from build123d import *

# Parameters (mm, degrees)
F1_DEPTH = 10
F2_START = 10
F2_DEPTH = 10
F3_START = 20
F3_DEPTH = 15
F4_START = 35
F4_DEPTH = 20


with BuildPart() as f1:
    # F0 (on Front) → F1 (new body)
    with BuildSketch(Plane.XZ):
        with BuildLine():
            Line((1.12e-08, 3), (-35, 3))
            Line((-35, 3), (-35, 0.5))
            Line((-35, 0.5), (-2.9580398915, 0.5))
            ThreePointArc((-2.9580398915, 0.5), (-1.9364916688, 2.2912878511), (1.12e-08, 3))
        make_face()
        with BuildLine():
            Line((-2.9580398915, 0.5), (-35, 0.5))
            Line((-35, 0.5), (-35, -0.5))
            Line((-35, -0.5), (-2.9580398915, -0.5))
            ThreePointArc((-2.9580398915, -0.5), (-3, 0), (-2.9580398915, 0.5))
        make_face()
        with BuildLine():
            Line((-2.9580398915, -0.5), (-35, -0.5))
            Line((-35, -0.5), (-35, -3))
            Line((-35, -3), (1.44e-08, -3))
            ThreePointArc((1.44e-08, -3), (-1.9364916676, -2.2912878521), (-2.9580398915, -0.5))
        make_face()
        with BuildLine():
            Line((2.9580398915, -0.5), (-2.9580398915, -0.5))
            ThreePointArc((-2.9580398915, -0.5), (-1.9364916676, -2.2912878521), (1.44e-08, -3))
            ThreePointArc((1.44e-08, -3), (1.9364916786, -2.2912878428), (2.9580398915, -0.5))
        make_face()
        with BuildLine():
            ThreePointArc((2.9580398915, 0.5), (1.9364916774, 2.2912878439), (1.12e-08, 3))
            ThreePointArc((1.12e-08, 3), (-1.9364916688, 2.2912878511), (-2.9580398915, 0.5))
            Line((-2.9580398915, 0.5), (2.9580398915, 0.5))
        make_face()
        with BuildLine():
            Line((35, 3), (1.12e-08, 3))
            ThreePointArc((1.12e-08, 3), (1.9364916774, 2.2912878439), (2.9580398915, 0.5))
            Line((2.9580398915, 0.5), (35, 0.5))
            Line((35, 0.5), (35, 3))
        make_face()
        with BuildLine():
            Line((35, 0.5), (2.9580398915, 0.5))
            ThreePointArc((2.9580398915, 0.5), (2.9894915684, 0.2508787808), (3, 0))
            ThreePointArc((3, 0), (2.9894915684, -0.2508787808), (2.9580398915, -0.5))
            Line((2.9580398915, -0.5), (35, -0.5))
            Line((35, -0.5), (35, 0.5))
        make_face()
        with BuildLine():
            Line((35, -3), (35, -0.5))
            Line((35, -0.5), (2.9580398915, -0.5))
            ThreePointArc((2.9580398915, -0.5), (1.9364916786, -2.2912878428), (1.44e-08, -3))
            Line((1.44e-08, -3), (35, -3))
        make_face()
        with BuildLine():
            ThreePointArc((3, 0), (2.9894915684, 0.2508787808), (2.9580398915, 0.5))
            Line((2.9580398915, 0.5), (-2.9580398915, 0.5))
            ThreePointArc((-2.9580398915, 0.5), (-3, 0), (-2.9580398915, -0.5))
            Line((-2.9580398915, -0.5), (2.9580398915, -0.5))
            ThreePointArc((2.9580398915, -0.5), (2.9894915684, -0.2508787808), (3, 0))
        make_face()
    extrude(amount=F1_DEPTH)

    # F0 (on Front) → F2 (join)
    with BuildSketch(Plane.XZ.offset(F2_START)):
        with BuildLine():
            Line((-2.9580398915, 0.5), (-35, 0.5))
            Line((-35, 0.5), (-35, -0.5))
            Line((-35, -0.5), (-2.9580398915, -0.5))
            ThreePointArc((-2.9580398915, -0.5), (-3, 0), (-2.9580398915, 0.5))
        make_face()
        with BuildLine():
            ThreePointArc((3, 0), (2.9894915684, 0.2508787808), (2.9580398915, 0.5))
            Line((2.9580398915, 0.5), (-2.9580398915, 0.5))
            ThreePointArc((-2.9580398915, 0.5), (-3, 0), (-2.9580398915, -0.5))
            Line((-2.9580398915, -0.5), (2.9580398915, -0.5))
            ThreePointArc((2.9580398915, -0.5), (2.9894915684, -0.2508787808), (3, 0))
        make_face()
        with BuildLine():
            Line((35, 0.5), (2.9580398915, 0.5))
            ThreePointArc((2.9580398915, 0.5), (2.9894915684, 0.2508787808), (3, 0))
            ThreePointArc((3, 0), (2.9894915684, -0.2508787808), (2.9580398915, -0.5))
            Line((2.9580398915, -0.5), (35, -0.5))
            Line((35, -0.5), (35, 0.5))
        make_face()
    extrude(amount=F2_DEPTH)

    # F0 (on Front) → F3 (join)
    with BuildSketch(Plane.XZ.offset(F3_START)):
        with BuildLine():
            Line((35, 3), (1.12e-08, 3))
            ThreePointArc((1.12e-08, 3), (1.9364916774, 2.2912878439), (2.9580398915, 0.5))
            Line((2.9580398915, 0.5), (35, 0.5))
            Line((35, 0.5), (35, 3))
        make_face()
        with BuildLine():
            Line((35, 0.5), (2.9580398915, 0.5))
            ThreePointArc((2.9580398915, 0.5), (2.9894915684, 0.2508787808), (3, 0))
            ThreePointArc((3, 0), (2.9894915684, -0.2508787808), (2.9580398915, -0.5))
            Line((2.9580398915, -0.5), (35, -0.5))
            Line((35, -0.5), (35, 0.5))
        make_face()
        with BuildLine():
            Line((35, -3), (35, -0.5))
            Line((35, -0.5), (2.9580398915, -0.5))
            ThreePointArc((2.9580398915, -0.5), (1.9364916786, -2.2912878428), (1.44e-08, -3))
            Line((1.44e-08, -3), (35, -3))
        make_face()
        with BuildLine():
            Line((-2.9580398915, -0.5), (-35, -0.5))
            Line((-35, -0.5), (-35, -3))
            Line((-35, -3), (1.44e-08, -3))
            ThreePointArc((1.44e-08, -3), (-1.9364916676, -2.2912878521), (-2.9580398915, -0.5))
        make_face()
        with BuildLine():
            Line((1.12e-08, 3), (-35, 3))
            Line((-35, 3), (-35, 0.5))
            Line((-35, 0.5), (-2.9580398915, 0.5))
            ThreePointArc((-2.9580398915, 0.5), (-1.9364916688, 2.2912878511), (1.12e-08, 3))
        make_face()
        with BuildLine():
            Line((-2.9580398915, 0.5), (-35, 0.5))
            Line((-35, 0.5), (-35, -0.5))
            Line((-35, -0.5), (-2.9580398915, -0.5))
            ThreePointArc((-2.9580398915, -0.5), (-3, 0), (-2.9580398915, 0.5))
        make_face()
        with BuildLine():
            ThreePointArc((2.9580398915, 0.5), (1.9364916774, 2.2912878439), (1.12e-08, 3))
            ThreePointArc((1.12e-08, 3), (-1.9364916688, 2.2912878511), (-2.9580398915, 0.5))
            Line((-2.9580398915, 0.5), (2.9580398915, 0.5))
        make_face()
        with BuildLine():
            ThreePointArc((3, 0), (2.9894915684, 0.2508787808), (2.9580398915, 0.5))
            Line((2.9580398915, 0.5), (-2.9580398915, 0.5))
            ThreePointArc((-2.9580398915, 0.5), (-3, 0), (-2.9580398915, -0.5))
            Line((-2.9580398915, -0.5), (2.9580398915, -0.5))
            ThreePointArc((2.9580398915, -0.5), (2.9894915684, -0.2508787808), (3, 0))
        make_face()
        with BuildLine():
            Line((2.9580398915, -0.5), (-2.9580398915, -0.5))
            ThreePointArc((-2.9580398915, -0.5), (-1.9364916676, -2.2912878521), (1.44e-08, -3))
            ThreePointArc((1.44e-08, -3), (1.9364916786, -2.2912878428), (2.9580398915, -0.5))
        make_face()
    extrude(amount=F3_DEPTH)

    # F0 (on Front) → F4 (join)
    with BuildSketch(Plane.XZ.offset(F4_START)):
        with BuildLine():
            Line((2.9580398915, -0.5), (-2.9580398915, -0.5))
            ThreePointArc((-2.9580398915, -0.5), (-1.9364916676, -2.2912878521), (1.44e-08, -3))
            ThreePointArc((1.44e-08, -3), (1.9364916786, -2.2912878428), (2.9580398915, -0.5))
        make_face()
        with BuildLine():
            ThreePointArc((3, 0), (2.9894915684, 0.2508787808), (2.9580398915, 0.5))
            Line((2.9580398915, 0.5), (-2.9580398915, 0.5))
            ThreePointArc((-2.9580398915, 0.5), (-3, 0), (-2.9580398915, -0.5))
            Line((-2.9580398915, -0.5), (2.9580398915, -0.5))
            ThreePointArc((2.9580398915, -0.5), (2.9894915684, -0.2508787808), (3, 0))
        make_face()
        with BuildLine():
            ThreePointArc((2.9580398915, 0.5), (1.9364916774, 2.2912878439), (1.12e-08, 3))
            ThreePointArc((1.12e-08, 3), (-1.9364916688, 2.2912878511), (-2.9580398915, 0.5))
            Line((-2.9580398915, 0.5), (2.9580398915, 0.5))
        make_face()
    extrude(amount=F4_DEPTH)


solid = f1.part
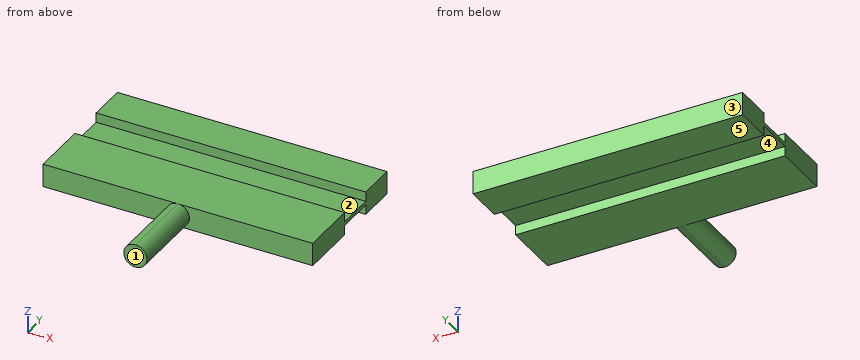
Verification items for the finished model (mm, model axes). Face numbers are marked on the shaded views. A direction names the side the tool comes from. Round coordinates to 2 decimals unless told otherwise and drop trailing zeros. Write each loop counter-clockwise with the first axis right and the second up, starting at its lowest first coordinate (ties: lowest second). Pieces come first, ordered by that corner, then holes.
(1) Depth check by flat-ended pin: pin 1 Ø1.2 at (x, z) = (-14.5, 1.5) entering from -Y; pin 2 Ø5 at (x, y) = (9.5, -13.5) entering from +Z; pin 3 Ø1 at (y, z) = (-36, -0.5) entering from +X. Enter the tip coordinate at first touch or a pass-through.
Returned:
pin 1: stops at y = -35
pin 2: stops at z = 0.5
pin 3: stops at x = 3
(2) Section check A-A (z = 1.8). Enter the section's corners in (x, y), plus the area to 3 significant figures.
Returned:
outline: (-35, -35) - (-2.4, -35) - (-2.4, -55) - (2.4, -55) - (2.4, -35) - (35, -35) - (35, -20) - (-35, -20) - close; (-35, -10) - (35, -10) - (35, 0) - (-35, 0) - close
area: 1,850 mm2
(3) Section check C-C (y = -37). Enter the section's corners in (x, z).
Returned:
outline: circle Ø6 at (0, 0)
(4) Material ranges on line 1 (Y direction, x = -18, z = 1.4); line 2 (Y direction, x = 0, z = 1.25); line 3 (Z direction, x = -8, y = -17), recorded low to high.
Returned:
line 1: y = -35 to -20, -10 to 0
line 2: y = -55 to -20, -10 to 0
line 3: z = -0.5 to 0.5
(5) Section check D-D (z = -1.95). Enter the section's corners in (x, y).
Returned:
outline: (-35, -35) - (-2.28, -35) - (-2.28, -55) - (2.28, -55) - (2.28, -35) - (35, -35) - (35, -20) - (-35, -20) - close; (-35, -10) - (35, -10) - (35, 0) - (-35, 0) - close
(6) Mould release check, pull along Y, two halves, no side actions. Record for the marked faces 3, 4 and 5: pulls with the +Y half, pulls with the -Y half, needs draft (parallel to the pull), parting line crosses it, or undercut.
Returned:
face 3: pulls with the +Y half
face 4: undercut
face 5: needs draft
(7) Section check B-B (x = -19.5). Enter the section's corners in (y, z).
Returned:
outline: (-35, -3) - (-20, -3) - (-20, -0.5) - (-10, -0.5) - (-10, -3) - (0, -3) - (0, 3) - (-10, 3) - (-10, 0.5) - (-20, 0.5) - (-20, 3) - (-35, 3) - close
(8) Access from +Z, -Z, +X, -X, +Y, -Y to the whole of each face (thin tool, end or side, straight path). Record for the marked faces 1 and 2.
Returned:
face 1: +Z, -Z, +X, -X, -Y
face 2: +Z, +X, -X
